Model file for the job. Use its own axes, mm. A direction names the side the tool comes from. Give positions to 0.01 mm unless a question says otherwise; leave off trailing zeros. Order: outer loops, then holes, each group sorted by start corner. A loop starts at its lowest first (then second) coordinate and runs counter-clockwise, first axis right, second up. Notation, with made-up numbers: (34, -40) - (59, -40) arc R14 ccw to (59, -18) - close; hole circle Ø9 at (56.5, 76). An arc over 180 degrees is marked (long way). Use CSV: the item, a comma, the result in double quotes. Start each with the question number.
(1) Probe L1, parallel to X at y = 7, z = 23 (3 decimals); L2, parallel to X at y = -14, z = 9 (3 decimals). List the from-to ranges inside material, lowest first.
(2) Drop flat-ended pins along their axis: pin 1 Ø7.5 at (y, z) = (0, 53.975) entering from +X (3 decimals); pin 2 Ø11 at (x, y) = (-27.5, 8) entering from +Z; pin 3 Ø10 at (x, z) = (0, 56) entering from +Y; pin 4 Ø1 at (y, z) = (-6, 37) entering from -X (3 decimals). Give the stop position or say it passes through.
(3) Band-saw the part on B-B, the plane y = 0. Count the separate pieces of the cut face and the enclosed holes in it, then the cut area to 3 significant figures.
(4) Tool access for faces 4 (the flat face through (-9.525, 0, 36)), 5 (the flat face through (21, 0, 4.762)), 6 (the cylindrical face through (-5.4, -0.3, 13.6)): list every direction of +Z, -Z, +X, -X, +Y, -Y with a clear straight run to the whole face (end or side of a thin tool).
(5) Band-saw the part on A-A, the plane z = 30. Give the cut face in (x, y) (3 decimals), then the cut area to 3 significant figures.
(6) Band-saw the part on D-D, the plane x = 16.5. Give the cut face in (y, z), then the cut area to 3 significant figures.
(7) Pull direction Y, two halves, no side cores. Call faces 1 (the flat face through (-8, 0, 63.5)), 2 (the cylindrical face through (7.92, 18.15, 62.55)), 3 (the cylindrical face through (23.165, -0.954, 2.348)): +Y half, -Y half, draft (parallel to the pull), parting line (faces both ways), or undercut.
from build123d import *

# Parameters (mm, degrees)
EXTRUDE1_DEPTH      = 19.05
SKETCH2_R           = 3.175
EXTRUDE2_DEPTH      = 75.93269063
EXTRUDE3_DEPTH      = 76.501141892
EXTRUDE3_DEPTH_BACK = 76.501141892
SKETCH3_R           = 3.175
FILLET3_R           = 3.1623


with BuildPart() as part:
    # Sketch1 → Extrude1 (new, symmetric)
    with BuildSketch(Plane(origin=(0, 0, 0), x_dir=(1, 0, 0), z_dir=(0, 1, 0))):
        Polygon((-34.925, 0), (34.925, 0), (34.925, -4.7625), (9.525, -4.7625), (9.525, -63.5), (6.35, -63.5), (6.35, -12.7), (-6.35, -12.7), (-6.35, -63.5), (-9.525, -63.5), (-9.525, -4.7625), (-34.925, -4.7625), align=None)
    extrude(amount=EXTRUDE1_DEPTH, both=True)

    # Sketch2 → Extrude2 (cut, through all)
    with BuildSketch(Plane.XY):
        with Locations(Location((-26.19375, 0, 0), (0, 0, 180))):
            Circle(SKETCH2_R)
        with Locations(Location((26.19375, 0, 0), (0, 0, 180))):
            Circle(SKETCH2_R)
    extrude(amount=EXTRUDE2_DEPTH, mode=Mode.SUBTRACT)

    # Sketch3 → Extrude3 (cut, two sides: drawn at the far end of the back side and taken through both)
    with BuildSketch(Plane(origin=(0, 0, -0.669808337), x_dir=(0, 0, -1), z_dir=(1, 0, 0)).offset(-EXTRUDE3_DEPTH_BACK)):
        with Locations(Location((-54.644808337, 0, 0), (0, 0, 180))):
            Circle(SKETCH3_R)
    extrude(amount=EXTRUDE3_DEPTH + EXTRUDE3_DEPTH_BACK, mode=Mode.SUBTRACT)

    # Fillet3
    fillet3_edges = [part.edges().sort_by_distance(p)[0] for p in [
        (-34.925, 19.05, 2.38125),
        (7.9375, -19.05, 63.5),
        (-7.9375, -19.05, 63.5),
        (-34.925, -19.05, 2.38125),
        (34.925, -19.05, 2.38125),
        (-7.9375, 19.05, 63.5),
        (9.525, 0, 4.7625),
        (6.35, 0, 12.7),
        (-6.35, 0, 12.7),
        (-9.525, 0, 4.7625),
        (7.9375, 19.05, 63.5),
        (34.925, 19.05, 2.38125),
    ]]
    fillet(fillet3_edges, radius=FILLET3_R)


solid = part.part
Answer block:
1,L1,"x = -9.525 to -6.35, 6.35 to 9.525"
1,L2,"x = -9.525 to 9.525"
2,pin 1,"stops at x = 9.525"
2,pin 2,"stops at z = 4.76"
2,pin 3,"passes through"
2,pin 4,"stops at x = -9.525"
3,separate pieces,"5"
3,enclosed holes,"0"
3,area,"714 mm2"
4,face 4,"+Z, -X, +Y, -Y"
4,face 5,"+Z, +X, +Y, -Y"
4,face 6,"+Z, +Y, -Y"
5,outline,"(-9.525, -19.05) - (-6.35, -19.05) - (-6.35, 19.05) - (-9.525, 19.05) - close; (6.35, -19.05) - (9.525, -19.05) - (9.525, 19.05) - (6.35, 19.05) - close"
5,area,"242 mm2"
6,outline,"(-19.05, 0) - (19.05, 0) - (19.05, 4.76) - (-19.05, 4.76) - close"
6,area,"181 mm2"
7,face 1,"draft"
7,face 2,"+Y half"
7,face 3,"undercut"
